```python
from build123d import *

# Parameters (mm, degrees)
F1_DEPTH = 12.7
F2_R     = 6.35
F3_R     = 3.175


with BuildPart() as f1:
    # F0 (on Front) → F1 (new body, symmetric)
    with BuildSketch(Plane.XZ):
        Polygon((-25.4, 0), (25.4, 0), (25.4, 12.7), (12.842343, 18.521002), (3.175, 31.75), (0.508, 31.75), (0.508, 12.7), (-0.508, 12.7), (-0.508, 31.75), (-3.175, 31.75), (-12.842343, 18.521002), (-25.4, 12.7), align=None)
    extrude(amount=F1_DEPTH, both=True)

    # F2
    f2_edges = [f1.edges().sort_by_distance(p)[0] for p in [
        (25.4, 0, 12.7),
        (12.842343, 0, 18.521002),
        (-12.842343, 0, 18.521002),
        (-25.4, 0, 12.7),
    ]]
    fillet(f2_edges, radius=F2_R)

    # F3
    f3_edges = [f1.edges().sort_by_distance(p)[0] for p in [
        (3.175, 0, 31.75),
        (-3.175, 0, 31.75),
    ]]
    fillet(f3_edges, radius=F3_R)


solid = f1.part
```
For this review, take the finished solid that the model builds, in its own axes (mm). A direction names the side the tool comes from. Round coordinates to 2 decimals unless told otherwise and drop trailing zeros. Write each loop counter-clockwise with the first axis right and the second up, starting at its lowest first coordinate (ties: lowest second). Pieces come first, ordered by that corner, then holes. Notation, with made-up numbers: (36, 56) -> (81, 56) arc R29 cw to (81, 94) -> close; hole circle Ø9 at (13.5, 5.25). An arc over 180 degrees is marked (long way). Use one line per item in the form item = value.
Q1. Machinability: for faces 4 (the flat face through (0.508, 0, 22)), 5 (the flat face through (8.055, -0.178, 25.073)), which of the approach directions +Z, -Z, +X, -X, +Y, -Y give a long, thin tool a straight path to every point of the face, cutting with its end or side? Answer none if there is none.
Resolved:
face_4 = +Z, +Y, -Y
face_5 = +Z, +X, +Y, -Y
Q2. The part is to be moulded in two halves that separate along X. For faces 1 (the flat face through (0, 0, 12.7)), 2 (the flat face through (25.4, 0, 4)), 3 (the cylindrical face through (-3.019, -0.178, 31.396)), say which applies: released by +X, released by -X, zero draft, split by the parting line, or undercut.
Resolved:
face_1 = undercut
face_2 = released by +X
face_3 = released by -X
Q3. Consider section C-C (x = -6.5). State the section outline as (y, z) points, then the cut area to 3 significant figures.
Resolved:
outline = (-12.7, 0) -> (12.7, 0) -> (12.7, 27.2) -> (-12.7, 27.2) -> close
area = 691 mm²
Q4. To check wall thickness, follow probe 1 along X at (y, z) = (10.25, 20); probe 2 along X at (y, z) = (0.75, 22); probe 3 along Z at (x, y) = (11.5, -2.5). State the ranges of each line that lie inside material, in increasing order. Write a range as from..to.
Resolved:
probe_1 = -11.76..-0.51, 0.51..11.76
probe_2 = -10.3..-0.51, 0.51..10.3
probe_3 = 0..20.36
Q5. Consider section D-D (z = 25.5). State the section outline as (x, y) points.
Resolved:
outline = (-7.74, -12.7) -> (-0.51, -12.7) -> (-0.51, 12.7) -> (-7.74, 12.7) -> close; (0.51, -12.7) -> (7.74, -12.7) -> (7.74, 12.7) -> (0.51, 12.7) -> close
Q6. Clearance check with flat-ended pins moving along their axes: pin 1 Ø12 at (y, z) = (-4, 25) entering from -X; pin 2 Ø1.5 at (y, z) = (9, 22.5) entering from -X; pin 3 Ø15 at (y, z) = (-5.5, 19.5) entering from -X. State where each tip first meets the part, or that it passes through.
Resolved:
pin_1 = -12.62
pin_2 = -10.48
pin_3 = -24.44
Q7. Consider section B-B (y = -0.5). State the section outline as (x, z) points (3 decimals), then the cut area to 3 significant figures.
Resolved:
outline = (-25.4, 0) -> (25.4, 0) -> (25.4, 8.644) arc R6.35 ccw to (21.721, 14.406) -> (14.331, 17.831) arc R6.35 cw to (11.874, 19.846) -> (4.126, 30.448) arc R3.175 ccw to (1.563, 31.75) -> (0.508, 31.75) -> (0.508, 12.7) -> (-0.508, 12.7) -> (-0.508, 31.75) -> (-1.563, 31.75) arc R3.175 ccw to (-4.126, 30.448) -> (-11.874, 19.846) arc R6.35 cw to (-14.331, 17.831) -> (-21.721, 14.406) arc R6.35 ccw to (-25.4, 8.644) -> close
area = 1,050 mm²
Q8. Consider section A-A (z = 16). State the section outline as (x, y) points, then the cut area to 3 significant figures.
Resolved:
outline = (-18.28, -12.7) -> (-0.51, -12.7) -> (-0.51, 12.7) -> (-18.28, 12.7) -> close; (0.51, -12.7) -> (18.28, -12.7) -> (18.28, 12.7) -> (0.51, 12.7) -> close
area = 903 mm²
